Geometry check sheet. Reference: the model listing, model coordinates, mm. Coordinates: 2 decimals unless noted, no trailing zeros. Order: outer loops, then holes, each group sorted by start corner. A loop starts at its lowest first (then second) coordinate and runs counter-clockwise, first axis right, second up. Notation, with made-up numbers: (25.5, -35.75) - (34.5, -35.75) arc R11 cw to (34.5, -23.75) - close; hole circle Ø5 at (-6, 89). An arc over 180 degrees is marked (long way). Put each result on its own line as item: value.
from build123d import *

# Parameters (mm, degrees)
SKETCH1_W           = 98.8568
SKETCH1_H           = 6.35
BOSS_EXTRUDE1_DEPTH = 6.35
SKETCH2_R           = 1.905
CUT_EXTRUDE1_DEPTH  = 116.667416004
SKETCH3_R           = 1.905
CUT_EXTRUDE2_DEPTH  = 105.09694142


with BuildPart() as part:
    # Sketch1 → Boss-Extrude1 (new body)
    with BuildSketch(Plane.XY):
        with Locations((-54.280462751, 47.649210884)):
            Rectangle(SKETCH1_W, SKETCH1_H)
    extrude(amount=BOSS_EXTRUDE1_DEPTH)

    # Sketch2 → Cut-Extrude1 (cut, through all)
    with BuildSketch(Plane.XY.offset(6.35)):
        with Locations((-100.533862751, 47.649210884)):
            Circle(SKETCH2_R)
        with Locations((-8.027062751, 47.649210884)):
            Circle(SKETCH2_R)
    extrude(amount=-CUT_EXTRUDE1_DEPTH, mode=Mode.SUBTRACT)

    # Sketch3 → Cut-Extrude2 (cut, through all)
    with BuildSketch(Plane(origin=(0, 50.824210884, 0), x_dir=(1, 0, 0), z_dir=(0, 1, 0))):
        with Locations(Location((-71.933462751, -3.175, 0), (0, 0, 270))):
            Circle(SKETCH3_R)
        with Locations(Location((-36.627462751, -3.175, 0), (0, 0, 270))):
            Circle(SKETCH3_R)
    extrude(amount=-CUT_EXTRUDE2_DEPTH, mode=Mode.SUBTRACT)


solid = part.part
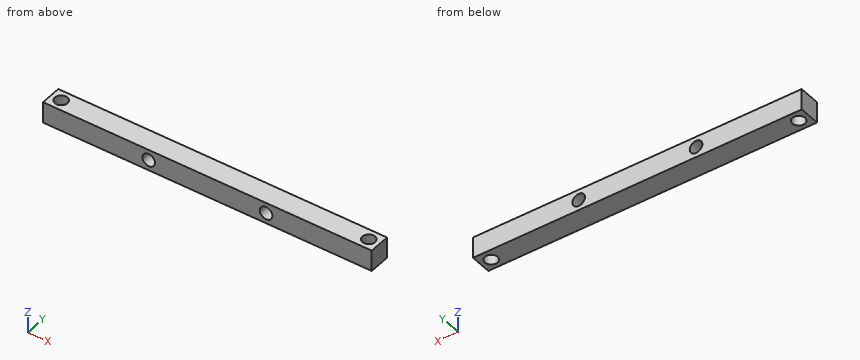
Q1. Section check B-B on z = 2.75. Record the boundary of the cut face in (x, y) (3 decimals), then the cut area to 3 significant figures.
Answer block:
outline: (-103.709, 44.474) - (-73.79, 44.474) - (-73.79, 50.824) - (-103.709, 50.824) - close; (-70.076, 44.474) - (-38.484, 44.474) - (-38.484, 50.824) - (-70.076, 50.824) - close; (-34.77, 44.474) - (-4.852, 44.474) - (-4.852, 50.824) - (-34.77, 50.824) - close; hole circle Ø3.81 at (-100.534, 47.649); hole circle Ø3.81 at (-8.027, 47.649)
area: 558 mm^2
Q2. Section check A-A on y = 46.75. Record the boundary of the cut face in (x, z) (3 decimals).
Answer block:
outline: (-103.709, 0) - (-102.213, 0) - (-102.213, 6.35) - (-103.709, 6.35) - close; (-98.854, 0) - (-9.706, 0) - (-9.706, 6.35) - (-98.854, 6.35) - close; (-6.348, 0) - (-4.852, 0) - (-4.852, 6.35) - (-6.348, 6.35) - close; hole circle Ø3.81 at (-71.933, 3.175); hole circle Ø3.81 at (-36.627, 3.175)
Q3. Thickness scan on L1, parallel to X at y = 48.75, z = 5.5; L2, parallel to X at y = 45.25, z = 2.25; L3, parallel to X at y = 47, z = 3.5. Record the ranges inside material, lowest first. Write a range as [from, to].
Answer block:
L1: x = [-103.71, -102.09], [-98.98, -9.58], [-6.47, -4.85]
L2: x = [-103.71, -73.6], [-70.27, -38.29], [-34.96, -4.85]
L3: x = [-103.71, -102.32], [-98.74, -73.81], [-70.06, -38.5], [-34.75, -9.82], [-6.24, -4.85]
